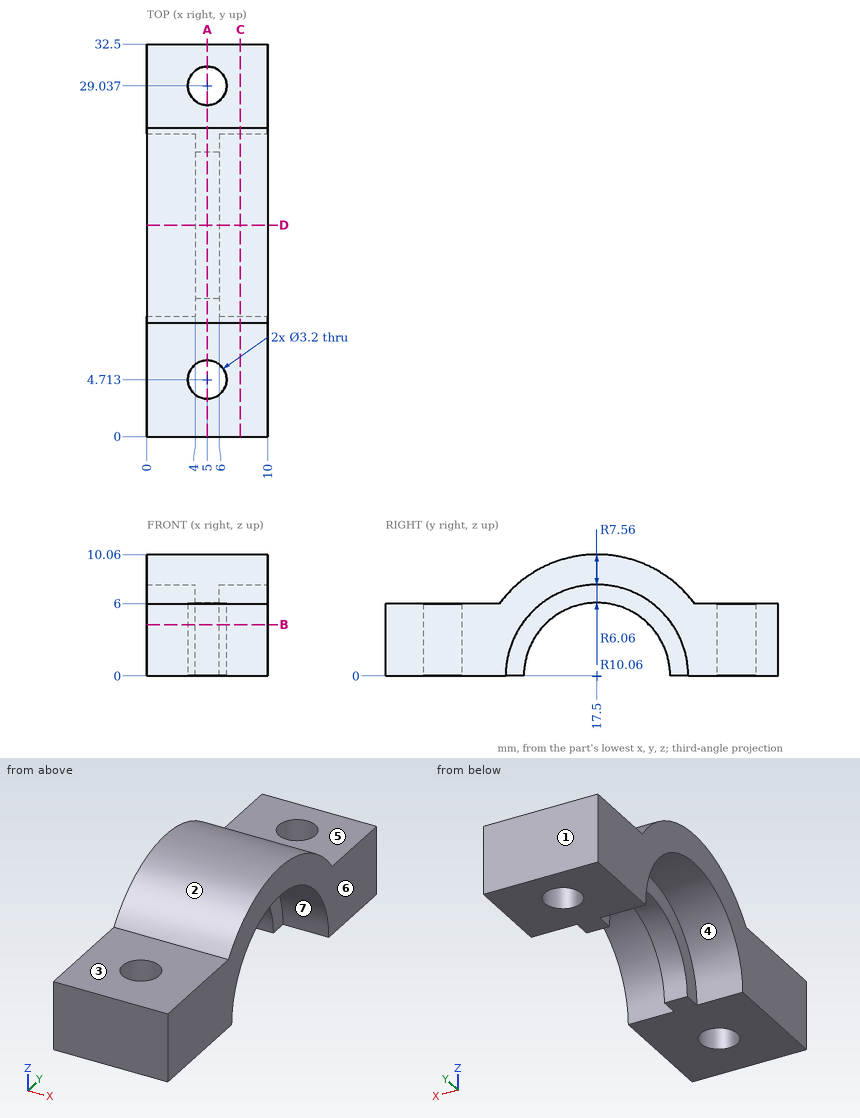
Design review of the part shown in the three views and the two pictorial views. Dimensions are in mm from the part's minimum x, y and z. A direction names the side the tool comes from. Give positions to 0.01 mm unless a question says otherwise; leave off trailing zeros. Order: outer loops, then holes, each group sorted by start corner. A loop starts at its lowest first (then second) coordinate and runs counter-clockwise, first axis right, second up. Notation, with made-up numbers: M 76.5,-19.5 L 116.5,-19.5 A20 ccw 116.5,-12.5 Z; hole C 81,69.5 d10. An arc over 180 degrees is marked long. Answer in a Markdown table with one row per item. Add a question column.
(1) Consider section B-B on z = 4.25. State the section outline as (x, y) points.
(2) Consider section D-D on y = 17.5. State the section outline as (x, z) points, and give its area (3 significant figures).
(3) Wall thickness on probe 1 along Y at (x, z) = (5, 2.75); probe 2 along Y at (x, z) = (6.25, 1) (1 decimal); probe 3 along X at (y, z) = (21.5, 5.75): over which ranges is each line inside the solid? List them lowest first. Write a range as [from, to].
(4) Consider section C-C on x = 7.75. State the section outline as (y, z) points (1 decimal), and give its area (3 significant figures).
(5) Consider section A-A on x = 5. State the section outline as (y, z) points (1 decimal), and give its area (3 significant figures).
(6) Mouldability with a two-part tool opening along Y and no side actions: class the marked faces 1, 2, 3 and 4 as +Y half, -Y half, draft (parallel to the pull), parting line (faces both ways), or undercut.
(7) For the marked faces 5, 6 and 7, list the 3-axis set-ups (+Z, -Z, +X, -X, +Y, -Y) from which the entire face can be reached by the end or side of a thin tool; tool diameter is ignored.
(8) For pin 1 (5.5 mm diameter, centred on x = 7, y = 29.5, fed in from +Z); pin 2 (4 mm diameter, centred on y = 17.5, z = 4.5, fed in from -X); pin 3 (3 mm diameter, centred on x = 2.5, y = 9.5, fed in from +Z), all flat-tipped, find the tip position at first contact; note any pin that passes through.
Evaluation:
| question | item | result |
|---|---|---|
| 1 | outline | M 0,0 L 10,0 L 10,11.25 L 6,11.25 L 6,13.18 L 4,13.18 L 4,11.25 L 0,11.25 Z; M 0,23.75 L 4,23.75 L 4,21.82 L 6,21.82 L 6,23.75 L 10,23.75 L 10,32.5 L 0,32.5 Z; hole C 5,4.71 d3.2; hole C 5,29.04 d3.2 |
| 2 | outline | M 0,7.56 L 4,7.56 L 4,6.06 L 6,6.06 L 6,7.56 L 10,7.56 L 10,10.06 L 0,10.06 Z |
| 2 | area | 28.0 mm^2 |
| 3 | probe 1 | y = [0, 3.11], [6.31, 12.1], [22.9, 27.44], [30.64, 32.5] |
| 3 | probe 2 | y = [0, 3.7], [5.7, 10], [25, 28], [30, 32.5] |
| 3 | probe 3 | x = [4, 6] |
| 4 | outline | M 0,0 L 9.9,0 A7.6 cw 25.1,0 L 32.5,0 L 32.5,6 L 25.6,6 A10.1 ccw 9.4,6 L 0,6 Z |
| 4 | area | 151 mm^2 |
| 5 | outline | M 0,0 L 3.1,0 L 3.1,6 L 0,6 Z; M 6.3,0 L 11.4,0 A6.1 cw 23.6,0 L 27.4,0 L 27.4,6 L 25.6,6 A10.1 ccw 9.4,6 L 6.3,6 Z; M 30.6,0 L 32.5,0 L 32.5,6 L 30.6,6 Z |
| 5 | area | 145 mm^2 |
| 6 | face 1 | +Y half |
| 6 | face 2 | parting line |
| 6 | face 3 | draft |
| 6 | face 4 | undercut |
| 7 | face 5 | +Z, +X, -X, +Y |
| 7 | face 6 | +Z, -Z, +X, +Y, -Y |
| 7 | face 7 | -Z, +X |
| 8 | pin 1 | stops at z = 6 |
| 8 | pin 2 | stops at x = 4 |
| 8 | pin 3 | stops at z = 7.68 |
